```python
from build123d import *

# Parameters (mm, degrees)
SKETCH1_R           = 1
BOSS_EXTRUDE1_DEPTH = 1.6
SKETCH2_W           = 59.5
SKETCH2_H           = 29.3
BOSS_EXTRUDE2_DEPTH = 1.2


with BuildPart() as part:
    # Sketch1 → Boss-Extrude1 (new body)
    with BuildSketch(Plane(origin=(0, 0, 0), x_dir=(1, 0, 0), z_dir=(0, 1, 0))):
        with BuildLine():
            Line((-33.145, -9.175), (-33.145, -16.375))
            ThreePointArc((-33.145, -16.375), (-32.559213562, -17.789213562), (-31.145, -18.375))
            Line((-31.145, -18.375), (31.145, -18.375))
            ThreePointArc((31.145, -18.375), (32.559213562, -17.789213562), (33.145, -16.375))
            Line((33.145, -16.375), (33.145, 16.375))
            ThreePointArc((33.145, 16.375), (32.559213562, 17.789213562), (31.145, 18.375))
            Line((31.145, 18.375), (-31.145, 18.375))
            ThreePointArc((-31.145, 18.375), (-32.559213562, 17.789213562), (-33.145, 16.375))
            Line((-33.145, 16.375), (-33.145, 9.975))
            Line((-33.145, 9.975), (-29.145, 9.975))
            Line((-29.145, 9.975), (-29.145, -9.175))
            Line((-29.145, -9.175), (-33.145, -9.175))
        make_face()
        with Locations(Location((-30.625, -16.125, 0), (0, 0, 270))):
            Circle(SKETCH1_R, mode=Mode.SUBTRACT)
        with Locations(Location((30.795, -16.125, 0), (0, 0, 270))):
            Circle(SKETCH1_R, mode=Mode.SUBTRACT)
        with Locations(Location((30.795, 16.225, 0), (0, 0, 270))):
            Circle(SKETCH1_R, mode=Mode.SUBTRACT)
        with Locations(Location((-30.625, 16.225, 0), (0, 0, 270))):
            Circle(SKETCH1_R, mode=Mode.SUBTRACT)
    extrude(amount=BOSS_EXTRUDE1_DEPTH)

    # Sketch2 → Boss-Extrude2 (add)
    with BuildSketch(Plane(origin=(0, 1.6, 0), x_dir=(1, 0, 0), z_dir=(0, 1, 0))):
        with Locations((2.895, -0.075)):
            Rectangle(SKETCH2_W, SKETCH2_H)
    extrude(amount=BOSS_EXTRUDE2_DEPTH)


solid = part.part
```
The model under review builds one solid part; all positions refer to its coordinate system, in mm. A direction names the side the tool comes from. Round coordinates to 2 decimals unless told otherwise and drop trailing zeros. Order: outer loops, then holes, each group sorted by start corner. A loop starts at its lowest first (then second) coordinate and runs counter-clockwise, first axis right, second up. Notation, with made-up numbers: M -34.75,-35.5 L 7.25,-35.5 A19 ccw 7.25,-10.5 Z; hole C 25.5,20 d9. An arc over 180 degrees is marked long. Use a Markdown table: item, result.
1) Wall thickness on line 1 along X through (y, z) = (1.2, -2.5) (3 decimals); line 2 along X through (y, z) = (1.95, -8) (3 decimals); line 3 along Z through (x, y) = (-8, 2.6) (3 decimals): over which ranges is each line inside the solid? List them lowest first. Write a range as [from, to].
Report:
| item | result |
|---|---|
| line 1 | [-29.145, 33.145] |
| line 2 | [-26.855, 32.645] |
| line 3 | [-14.575, 14.725] |
2) Insertion check: pin 1 (0.6 mm diameter, centred on y = 2, z = -4.5, fed in from -X) (3 decimals); pin 2 (0.5 mm diameter, centred on x = -31.5, y = 0.5, fed in from -Z); pin 3 (0.6 mm diameter, centred on x = -0.5, y = 2, fed in from +Z) (3 decimals); pin 4 (1.8 mm diameter, centred on x = 30.795, z = -16.225, fed in from +Y). Each pin has a flat end and moves straight along its axis. Give the tip position at first contact, or say it passes through.
Report:
| item | result |
|---|---|
| pin 1 | x = -26.855 |
| pin 2 | z = -18.37 |
| pin 3 | z = 14.725 |
| pin 4 | through |
3) Consider section C-C (y = 1.15). Write out the cut boundary in (x, z) (3 decimals), then the cut area to 3 significant figures.
Report:
| item | result |
|---|---|
| outline | M -33.145,-16.375 A2 ccw -31.145,-18.375 L 31.145,-18.375 A2 ccw 33.145,-16.375 L 33.145,16.375 A2 ccw 31.145,18.375 L -31.145,18.375 A2 ccw -33.145,16.375 L -33.145,9.175 L -29.145,9.175 L -29.145,-9.975 L -33.145,-9.975 Z; hole C -30.625,-16.225 d2; hole C -30.625,16.125 d2; hole C 30.795,-16.225 d2; hole C 30.795,16.125 d2 |
| area | 2,340 mm^2 |
4) Draft analysis for pull direction Z (two halves, no side actions). For faces 1 (the face through (32.544, 0.789, 17.805)), 2 (the face through (-5, 1.6, -15)), 3 (the face through (-29.634, 0.789, -16.355)), state which applies: released by +Z, released by -Z, zero draft, split by the parting line, or undercut.
Report:
| item | result |
|---|---|
| face 1 | released by +Z |
| face 2 | zero draft |
| face 3 | undercut |
5) Consider section A-A (x = 0). Write out the cut boundary in (y, z) (3 decimals).
Report:
| item | result |
|---|---|
| outline | M 0,-18.375 L 1.6,-18.375 L 1.6,-14.575 L 2.8,-14.575 L 2.8,14.725 L 1.6,14.725 L 1.6,18.375 L 0,18.375 Z |
6) Consider section B-B (z = 12.5). Write out the cut boundary in (x, y) (3 decimals), then the cut area to 3 significant figures.
Report:
| item | result |
|---|---|
| outline | M -33.145,0 L 33.145,0 L 33.145,1.6 L 32.645,1.6 L 32.645,2.8 L -26.855,2.8 L -26.855,1.6 L -33.145,1.6 Z |
| area | 177 mm^2 |
7) Tool access review of faces 4 (the face through (32.645, 2, 0)), 5 (the face through (-26.855, 2, 0)), 6 (the face through (-29.145, 1, -1)), 7 (the face through (2, 2, -14.575)): name each direction out of +Z, -Z, +X, -X, +Y, -Y from which nothing blocks a thin tool from reaching the whole face with its end or side.
Report:
| item | result |
|---|---|
| face 4 | +Z, -Z, +X, +Y |
| face 5 | +Z, -Z, -X, +Y |
| face 6 | -X, +Y, -Y |
| face 7 | -Z, +X, -X, +Y |
